Design review of the part built by this model. Coordinates are the model's own, in mm. A direction names the side the tool comes from. Coordinates: 2 decimals unless noted, no trailing zeros. Write each loop counter-clockwise with the first axis right and the second up, starting at its lowest first coordinate (ties: lowest second). Pieces come first, ordered by that corner, then holes. Notation, with made-up numbers: M 56.25,-14.75 L 63.25,-14.75 A21 ccw 63.25,4.25 Z; hole C 62.5,38.25 d6. An arc over 180 degrees is marked long. Write item = value, one per line.
```python
from build123d import *

# Parameters (mm, degrees)
SKETCH1_R           = 2.718976156
BOSS_EXTRUDE1_DEPTH = 5


with BuildPart() as part:
    # Sketch1 → Boss-Extrude1 (new body, symmetric)
    with BuildSketch(Plane.XY):
        with BuildLine():
            Line((-71.230316372, 16.423183965), (-69.697125978, 14.874544766))
            ThreePointArc((-69.697125978, 14.874544766), (-70.178618015, 14.345414894), (-70.602445452, 13.769061439))
            Line((-70.602445452, 13.769061439), (-72.282613853, 14.874544766))
            Line((-72.282613853, 14.874544766), (-73.429019542, 13.132180531))
            Line((-73.429019542, 13.132180531), (-71.477844105, 11.848385459))
            ThreePointArc((-71.477844105, 11.848385459), (-71.668751879, 10.930245938), (-71.732785885, 9.994657565))
            Line((-71.732785885, 9.994657565), (-73.852173913, 9.994657565))
            Line((-73.852173913, 9.994657565), (-73.852173913, 7.904409303))
            Line((-73.852173913, 7.904409303), (-71.406922201, 7.904409303))
            ThreePointArc((-71.406922201, 7.904409303), (-71.290285788, 7.56950355), (-71.156514693, 7.24106602))
            Line((-71.156514693, 7.24106602), (-86.578147363, -6.260758332))
            Line((-86.578147363, -6.260758332), (-82.977208325, -9.89798132))
            Line((-82.977208325, -9.89798132), (-67.353165307, 3.488554168))
            Line((-67.353165307, 3.488554168), (-68.096179637, 1.544987721))
            ThreePointArc((-68.096179637, 1.544987721), (-66.508347558, 1.098932073), (-64.865919209, 0.948580907))
            Line((-64.865919209, 0.948580907), (-64.865919209, 3.127790889))
            ThreePointArc((-64.865919209, 3.127790889), (-63.601066667, 3.24528678), (-62.37949878, 3.593753614))
            Line((-62.37949878, 3.593753614), (-61.590429693, 1.562417569))
            ThreePointArc((-61.590429693, 1.562417569), (-60.160877534, 2.268462787), (-58.877488851, 3.214524472))
            Line((-58.877488851, 3.214524472), (-60.320108421, 4.847866116))
            ThreePointArc((-60.320108421, 4.847866116), (-59.523604951, 5.680316792), (-58.877488851, 6.634217149))
            Line((-58.877488851, 6.634217149), (-56.977051893, 5.567776566))
            ThreePointArc((-56.977051893, 5.567776566), (-56.570785994, 6.386019614), (-56.249119541, 7.24106602))
            Line((-56.249119541, 7.24106602), (-58.324916217, 7.904409303))
            ThreePointArc((-58.324916217, 7.904409303), (-58.144259528, 8.589969318), (-58.035251347, 9.290502395))
            Line((-58.035251347, 9.290502395), (-56.249119541, 9.290502395))
            Line((-56.249119541, 9.290502395), (-56.249119541, 10.916483695))
            Line((-56.249119541, 10.916483695), (-58.125115153, 10.916483695))
            Line((-58.125115153, 10.916483695), (-58.534150947, 12.652206929))
            Line((-58.534150947, 12.652206929), (-56.249119541, 13.611272945))
            Line((-56.249119541, 13.611272945), (-57.500945462, 15.156219029))
            Line((-57.500945462, 15.156219029), (-59.21291168, 13.769061439))
            Line((-59.21291168, 13.769061439), (-60.336886068, 15.156219029))
            Line((-60.336886068, 15.156219029), (-59.44992841, 17.136193302))
            Line((-59.44992841, 17.136193302), (-61.290349947, 18.148130182))
            Line((-61.290349947, 18.148130182), (-61.770458694, 16.124256422))
            Line((-61.770458694, 16.124256422), (-63.907050908, 16.794247959))
            Line((-63.907050908, 16.794247959), (-63.907050908, 18.989771489))
            Line((-63.907050908, 18.989771489), (-65.82478751, 18.989771489))
            Line((-65.82478751, 18.989771489), (-65.82478751, 16.794247959))
            Line((-65.82478751, 16.794247959), (-68.096179637, 16.054300748))
            Line((-68.096179637, 16.054300748), (-69.121307415, 17.977337199))
            Line((-69.121307415, 17.977337199), (-71.230316372, 16.423183965))
        make_face()
        with Locations((-64.865919209, 9.994657565)):
            Circle(SKETCH1_R, mode=Mode.SUBTRACT)
    extrude(amount=BOSS_EXTRUDE1_DEPTH, both=True)


solid = part.part
```
Q1. The part is to be moulded in two halves that separate along Y. For faces 6 (the cylindrical face through (-71.667, 10.943, 0.07)), 7 (the flat face through (-58.345, 14.472, 0.07)), 8 (the flat face through (-73, 7.904, 0)), 9 (the flat face through (-69, 5, -5)), say which applies: +Y half, -Y half, draft (parallel to the pull), parting line (faces both ways), or undercut.
Check result:
face_6 = undercut
face_7 = +Y half
face_8 = undercut
face_9 = draft
Q2. Wall thickness on line 1 (Y direction, x = -58, z = 1); line 2 (Y direction, x = -73, z = 1.5); line 3 (X direction, y = 10.25, z = 2.5): over which ranges is each line inside the solid? List them lowest first.
Check result:
line_1 = 6.14 to 7.8, 9.29 to 10.92, 12.88 to 14.75
line_2 = -1.35 to 5.63, 7.9 to 9.99, 12.85 to 13.78
line_3 = -71.73 to -67.57, -62.16 to -56.25
Q3. Consider section D-D, the plane y = -7. State the section outline as (x, z) points, and give its area (3 significant figures).
Check result:
outline = M -85.85,-5 L -79.59,-5 L -79.59,5 L -85.85,5 Z
area = 62.5 mm²
Q4. Consider section C-C, the plane x = -83.5. State the section outline as (y, z) points, and give its area (3 significant figures).
Check result:
outline = M -9.37,-5 L -3.57,-5 L -3.57,5 L -9.37,5 Z
area = 58.0 mm²
Q5. Consider section B-B, the plane y = 2. State the section outline as (x, z) points, and give its area (3 significant figures).
Check result:
outline = M -77.14,-5 L -69.09,-5 L -69.09,5 L -77.14,5 Z; M -67.92,-5 L -64.87,-5 L -64.87,5 L -67.92,5 Z; M -61.76,-5 L -60.63,-5 L -60.63,5 L -61.76,5 Z
area = 122 mm²
Q6. Consider section A-A, the plane y = 14.5. State the section outline as (x, z) points.
Check result:
outline = M -72.53,-5 L -71.71,-5 L -71.71,5 L -72.53,5 Z; M -70.05,-5 L -59.81,-5 L -59.81,5 L -70.05,5 Z; M -58.31,-5 L -56.97,-5 L -56.97,5 L -58.31,5 Z
Q7. Machinability: for faces 1 (the flat face through (-57, 10.916, 0)), 2 (the flat face through (-71.431, 14.314, 0.07)), 3 (the flat face through (-62.824, 16.455, 0.07)), 4 (the cylindrical face through (-66.531, 1.103, 0.07)), 5 (the flat face through (-73.852, 9, 0)), which of the approach directions +Z, -Z, +X, -X, +Y, -Y give a long, thin tool a straight path to every point of the face, cutting with its end or side? Answer none if there is none.
Check result:
face_1 = +Z, -Z, +X
face_2 = +Z, -Z
face_3 = +Z, -Z, +Y
face_4 = +Z, -Z, -Y
face_5 = +Z, -Z, -X, +Y
Q8. For P1, Ø1.5, axis at x = -57.5, z = -2, coming from the +Y side; P2, Ø5, axis at x = -64.5, z = -3.5, coming from the -Y side; P3, Ø2.5, axis at x = -73, z = 0, coming from the +Y side; P4, Ø1, axis at x = -76, y = -7, coming from the -Z side, all flat-tipped, find the tip position at first contact; note any pin that passes through.
Check result:
P1 = 15.16
P2 = 0.95
P3 = 14.87
P4 = through
